The listing builds one solid part. Answer for the finished solid, in the listing's coordinates (mm). Give positions to 0.01 mm unless a question says otherwise; leave off trailing zeros. Write each loop counter-clockwise with the first axis right and the second up, starting at its lowest first coordinate (ties: lowest second). Pieces come first, ordered by that corner, then holes. Notation, with made-up numbers: (9.5, -7.5) - (52.5, -7.5) arc R12 ccw to (52.5, 0.5) - close; hole circle Ø3 at (4.5, 69). An arc over 180 degrees is marked (long way). Return JSON: item names as keys, results as strings.
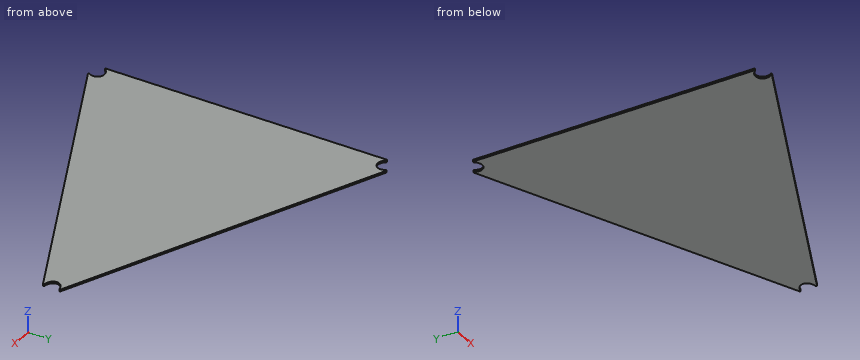
from build123d import *

# Parameters (mm, degrees)
BOSS_EXTRUDE1_DEPTH = 3.175
FILLET1_R           = 1.27


with BuildPart() as part:
    # Sketch2 → Boss-Extrude1 (new body)
    with BuildSketch(Plane.XY):
        with BuildLine():
            add(Edge.make_bspline(
                [(-224.002225489, 237.681676079), (-232.004852581, 227.466830346), (-248.536961255, 229.708235903), (-248.531511338, 247.553045118)],
                knots=[0, 0, 0, 0, 0.379035755, 0.379035755, 0.379035755, 0.379035755], degree=3, weights=[1, 0.494618994, 0.37235293, 0.633201808]))
            Line((-248.531511338, 247.553045118), (-248.68268269, -247.431362977))
            add(Edge.make_bspline(
                [(-248.68268269, -247.431362977), (-248.677234709, -229.592890963), (-232.152010305, -227.358084205), (-224.153396841, -237.567806796)],
                knots=[0.621058297, 0.621058297, 0.621058297, 0.621058297, 1, 1, 1, 1], degree=3, weights=[0.633007703, 0.37241363, 0.494744396, 1]))
            add(Edge.make_bspline(
                [(-224.153396841, -237.567806796), (-219.422565419, -243.606412946), (-220.040878469, -253.31787844), (-230.404432953, -258.064554967)],
                knots=[0, 0, 0, 0, 0.282425472, 0.282425472, 0.282425472, 0.282425472], degree=3, weights=[1, 0.623432704, 0.459569801, 0.50841129]))
            Line((-230.404432953, -258.064554967), (308.83327514, -11.084913444))
            add(Edge.make_bspline(
                [(308.83327514, -11.084913444), (295.43695815, -17.220644529), (285.763127193, -9.203898597), (285.763127193, 0)],
                knots=[0.684854095, 0.684854095, 0.684854095, 0.684854095, 1, 1, 1, 1], degree=3, weights=[0.533951912, 0.424456097, 0.57980546, 1]))
            add(Edge.make_bspline(
                [(285.763127193, 0), (285.763127193, 9.206022551), (295.440494393, 17.223574641), (308.837548746, 11.082955337)],
                knots=[0, 0, 0, 0, 0.315188067, 0.315188067, 0.315188067, 0.315188067], degree=3, weights=[1, 0.579749243, 0.424414534, 0.533995873]))
            Line((308.837548746, 11.082955337), (-230.249394824, 258.176652546))
            add(Edge.make_bspline(
                [(-230.249394824, 258.176652546), (-219.88947652, 253.42812256), (-219.272438092, 243.718949596), (-224.002225489, 237.681676079)],
                knots=[0.717613388, 0.717613388, 0.717613388, 0.717613388, 1, 1, 1, 1], degree=3, weights=[0.508391141, 0.459614898, 0.623484517, 1]))
        make_face()
    extrude(amount=BOSS_EXTRUDE1_DEPTH)

    # Fillet1
    fillet1_edges = [part.edges().sort_by_distance(p)[0] for p in [
        (-230.249394824, 258.176652546, 1.5875),
    ]]
    fillet(fillet1_edges, radius=FILLET1_R)
    fillet1_2_edges = [part.edges().sort_by_distance(p)[0] for p in [
        (-248.531511338, 247.553045118, 1.5875),
    ]]
    fillet(fillet1_2_edges, radius=FILLET1_R)
    fillet1_3_edges = [part.edges().sort_by_distance(p)[0] for p in [
        (-230.404432953, -258.064554967, 1.5875),
    ]]
    fillet(fillet1_3_edges, radius=FILLET1_R)
    fillet1_4_edges = [part.edges().sort_by_distance(p)[0] for p in [
        (308.837548746, 11.082955337, 1.5875),
    ]]
    fillet(fillet1_4_edges, radius=FILLET1_R)
    fillet1_5_edges = [part.edges().sort_by_distance(p)[0] for p in [
        (-248.68268269, -247.431362977, 1.5875),
    ]]
    fillet(fillet1_5_edges, radius=FILLET1_R)
    # the kernel refuses this fillet: 1.27 mm, written as the material it takes off along each edge
    with BuildSketch(Plane(origin=(308.833274988, -11.084913514, -23.853565642), x_dir=(-0.909173978372099, -0.4164164706769535, 0), z_dir=(0, 0, 1))) as fillet1_6_piece_1:
        with BuildLine():
            CenterArc((9.54142609, -1.27), FILLET1_R, 90, 150.734300738)
            Line((8.920573521, -2.377899855), (8.908156469, -2.400057852))
            ThreePointArc((8.908156469, -2.400057852), (4.606653366, -0.645600152), (0, -0.0254))
            Line((0, -0.0254), (0, 0.0254))
            Line((0, 0.0254), (9.54142609, 0.0254))
            Line((9.54142609, 0.0254), (9.54142609, 0))
        make_face()
    extrude(amount=50.882131284, mode=Mode.SUBTRACT)


solid = part.part
Item 1: Consider L1, parallel to X at y = 2.5, z = 0.9; L2, parallel to Y at x = -61.5, z = 1.4; L3, parallel to Y at x = -165, z = 2.65. Determine where each line is inside the solid, lowest interval first.
Answer below:
{"L1": "x = -248.61 to 286.07", "L2": "y = -180.7 to 180.83", "L3": "y = -228.11 to 228.27"}
Item 2: A flat-ended cylindrical pin translates along its axis: P1, Ø1, axis at y = -52.5, z = 1.5, coming from the -X side. Find the tip coordinate at first contact, or state that the pin passes through.
Answer below:
{"P1": "stops at x = -248.62"}
Item 3: A cutting plane is placed at A-A on x = -100. Determine the outline of the cut face in (y, z) (3 decimals), then the cut area to 3 significant figures.
Answer below:
{"outline": "(-198.337, 0) - (198.476, 0) - (198.476, 3.175) - (-198.337, 3.175) - close", "area": "1,260 mm²"}
Item 4: A cutting plane is placed at B-B on y = 160. Determine the outline of the cut face in (x, z) (3 decimals).
Answer below:
{"outline": "(-248.558, 0) - (-16.056, 0) - (-16.056, 3.175) - (-248.558, 3.175) - close"}
